The drawing under review shows one solid part. Ordinate dimensions are in mm from its lowest x, y, z. Give positions to 0.01 mm unless a question says otherwise; leave off trailing zeros. Write each loop counter-clockwise with the first axis right and the second up, starting at its lowest first coordinate (ties: lowest second). Pieces come first, ordered by that corner, then holes. Notation, with made-up numbers: M 61,81.5 L 70,81.5 A22 cw 70,92.5 Z; hole C 27.5,65 d6. An arc over 180 degrees is marked long. Use one line per item in the form item = value. Start each with the question number.
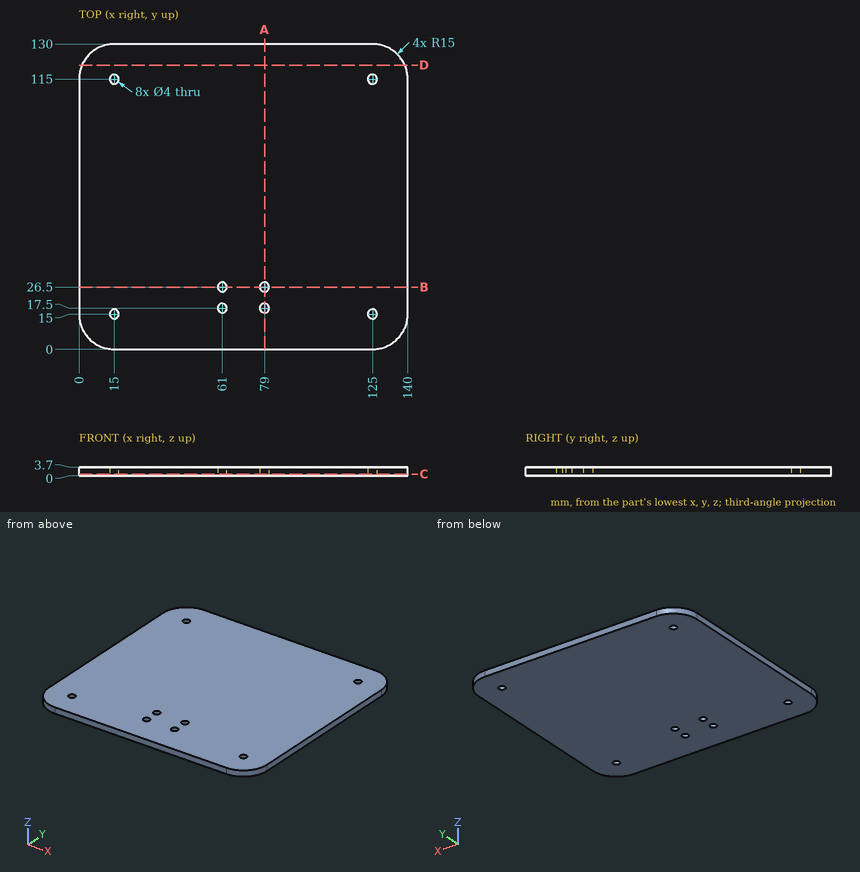
1. We need section B-B (y = 26.5). State the section outline as (x, z) points.
2. We need section D-D (y = 121). State the section outline as (x, z) points.
3. We need section A-A (x = 79). State the section outline as (y, z) points.
4. Clearance check with flat-ended pins moving along their axes: pin 1 Ø4.5 at (x, y) = (125, 115) entering from -Z; pin 2 Ø3.5 at (x, y) = (79, 17.5) entering from +Z. State where each tip first meets the part, or that it passes through.
5. We need section C-C (z = 0.8). Give the number of separate pieces and of enclosed holes in the cut face, and give its area (3 significant figures).
6. To check wall thickness, follow L1, parallel to Y at x = 15, z = 0.85; L2, parallel to Y at x = 61, z = 2.25; L3, parallel to X at y = 18, z = 1.3. State the ranges of each line that lie inside material, in increasing order.
Answer block:
q1.outline = M 0,0 L 59,0 L 59,3.7 L 0,3.7 Z; M 63,0 L 77,0 L 77,3.7 L 63,3.7 Z; M 81,0 L 140,0 L 140,3.7 L 81,3.7 Z
q2.outline = M 1.25,0 L 138.75,0 L 138.75,3.7 L 1.25,3.7 Z
q3.outline = M 0,0 L 15.5,0 L 15.5,3.7 L 0,3.7 Z; M 19.5,0 L 24.5,0 L 24.5,3.7 L 19.5,3.7 Z; M 28.5,0 L 130,0 L 130,3.7 L 28.5,3.7 Z
q4.pin_1 = 0
q4.pin_2 = through
q5.separate_pieces = 1
q5.enclosed_holes = 8
q5.area = 17,900 mm^2
q6.L1 = 0 to 13, 17 to 113, 117 to 130
q6.L2 = 0 to 15.5, 19.5 to 24.5, 28.5 to 130
q6.L3 = 0 to 59.06, 62.94 to 77.06, 80.94 to 140
